Answer from the drawing. Dimensions are ordinates in mm from the lowest x, y and z of the part. A direction names the side the tool comes from. Coordinates: 2 decimals unless noted, no trailing zeros. Order: outer loops, then holes, each group sorted by start corner. A loop starts at its lowest first (then second) coordinate and runs counter-clockwise, first axis right, second up. Notation, with made-up numbers: (85.25, -18) -> (100.25, -18) arc R31 ccw to (100.25, 19) -> close; hole circle Ø1 at (43.5, 48). An arc over 180 degrees is marked (long way). Answer as a JSON object with one key per item and string values. Group by question number.
1) A tool of negligible diameter and unlimited length cuts with its end or side. For the marked faces 1 and 2, from which of +Z, -Z, +X, -X, +Y, -Y can it reach the whole face along a straight path? Write none if from no direction.
2) Section B-B on y = 187 is taken. Determine the outline of the cut face in (x, z) (1 decimal).
3) Section C-C on x = 65 is taken. Determine the outline of the cut face in (y, z) (1 decimal).
4) Section A-A on z = 38.1 is taken. Determine the outline of the cut face in (x, y) (1 decimal), and give its area (3 significant figures).
5) Given pin 1 (3 mm diameter, centred on y = 395.5, z = 60, fed in from +X) (1 decimal); pin 2 (1 mm diameter, centred on x = 61.5, y = 457, fed in from +Z) (1 decimal); pin 3 (8.5 mm diameter, centred on y = 363.54, z = 38.1, fed in from +X); pin 4 (5 mm diameter, centred on x = 28, y = 70, fed in from -Z), each flat-ended and moving along its own axis, determine where each tip first touches the part or whether it passes through.
6) Consider L1, parallel to Y at x = 7, z = 38 (1 decimal); L2, parallel to Z at x = 36.5, y = 386.5 (1 decimal). Determine where each line is inside the solid, lowest interval first.
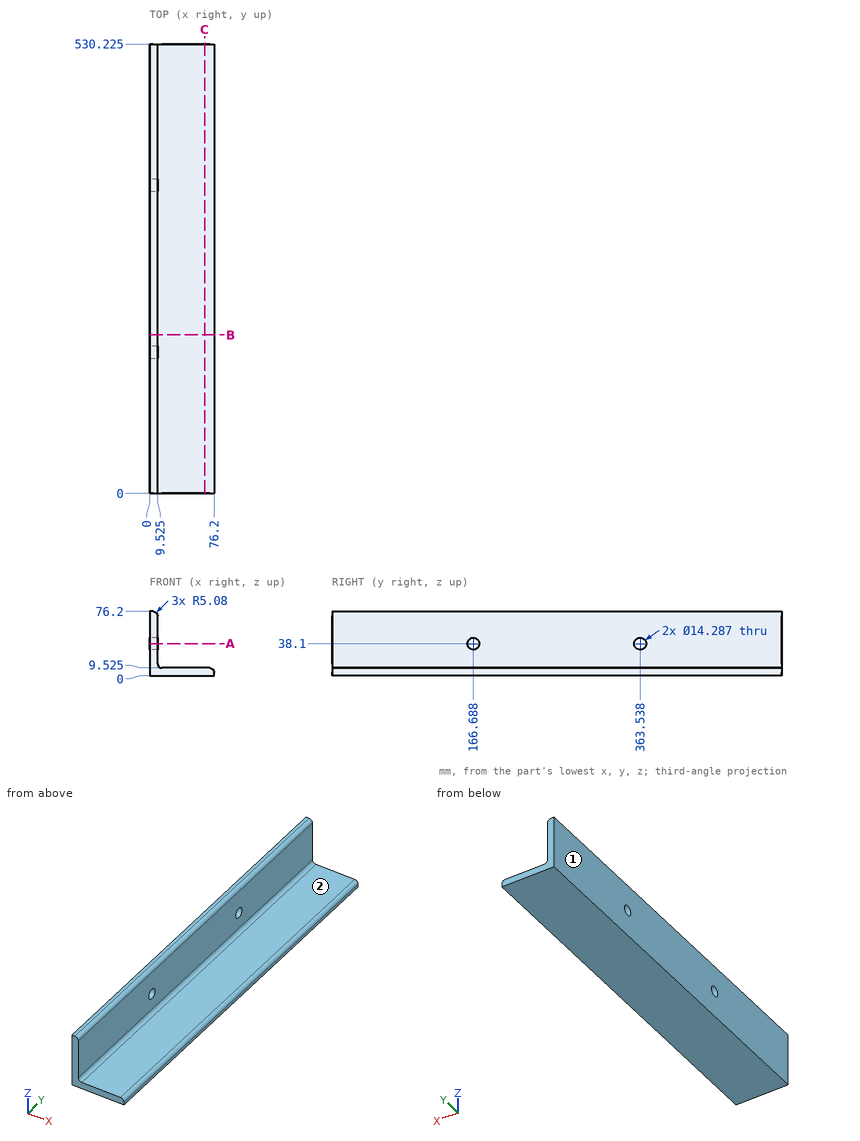
Worked answers:
{
 "1": {"face 1": "+Z, -Z, -X, +Y, -Y", "face 2": "+Z, +X, +Y, -Y"},
 "2": {"outline": "(0, 0) -> (76.2, 0) -> (76.2, 4.4) arc R5.1 ccw to (71.1, 9.5) -> (14.6, 9.5) arc R5.1 cw to (9.5, 14.6) -> (9.5, 71.1) arc R5.1 ccw to (4.4, 76.2) -> (0, 76.2) -> close"},
 "3": {"outline": "(0, 0) -> (530.2, 0) -> (530.2, 9.5) -> (0, 9.5) -> close"},
 "4": {"outline": "(0, 0) -> (9.5, 0) -> (9.5, 159.5) -> (0, 159.5) -> close; (0, 173.8) -> (9.5, 173.8) -> (9.5, 356.4) -> (0, 356.4) -> close; (0, 370.7) -> (9.5, 370.7) -> (9.5, 530.2) -> (0, 530.2) -> close", "area": "4,780 mm²"},
 "5": {"pin 1": "stops at x = 9.5", "pin 2": "stops at z = 9.5", "pin 3": "passes through", "pin 4": "stops at z = 0"},
 "6": {"L1": "y = 0 to 159.5, 173.8 to 356.4, 370.7 to 530.2", "L2": "z = 0 to 9.5"}
}
